Design review of the part built by this model. Coordinates are the model's own, in mm. Face numbers are marked on the shaded views. A direction names the side the tool comes from. Coordinates: 2 decimals unless noted, no trailing zeros. Loops run counter-clockwise (first coordinate to the right, second up) from the corner with the lowest first, then second, coordinate; pieces in that order, holes last. Notation, with made-up numbers: (60, 82) - (74, 82) arc R28 ccw to (74, 117) - close; hole circle Ø9 at (-34.75, -2). An arc over 180 degrees is marked (long way). Answer in a Markdown table with one row per item. Add a question column.
(1) We need section C-C, the plane z = -1.75. Write out the cut boundary in (x, y).
(2) We need section D-D, the plane x = 0. Write out the cut boundary in (y, z).
(3) The part is to be moulded in two halves that separate along Y. For the marked faces 3, 4, 5 and 6, say which applies: released by +Y, released by -Y, zero draft, split by the parting line, or undercut.
(4) We need section B-B, the plane x = -7.5. Write out the cut boundary in (y, z), plus the area to 3 significant figures.
(5) To check wall thickness, follow L1, parallel to Y at x = 24.5, z = -3; L2, parallel to X at y = -9.5, z = 2.75; L3, parallel to X at y = 12.5, z = 0. State the ranges of each line that lie inside material, in increasing order. Write a range as [from, to].
(6) Clearance check with a flat-ended pin moving along its axis: pin 1 (6.5 mm diameter, centred on x = 30, z = 0, fed in from -Y). State where the tip first meets the part, or that it passes through.
(7) For the marked faces 1 and 2, list the 3-axis set-ups (+Z, -Z, +X, -X, +Y, -Y) from which the entire face can be reached by the end or side of a thin tool; tool diameter is ignored.
(8) We need section A-A, the plane y = -4. Write out the cut boundary in (x, z), plus the area to 3 significant figures.
from build123d import *

# Parameters (mm, degrees)
F0_W          = 75
F0_H          = 50
F0_W_2        = 60
F0_H_2        = 40
F1_DEPTH      = 12.5
F2_R          = 2.5
F3_DEPTH      = 25.001
F3_DEPTH_BACK = 25.001


with BuildPart() as f1:
    # F0 (on Top) → F1 (new body, symmetric)
    with BuildSketch(Plane.XY):
        Rectangle(F0_W, F0_H)
        Rectangle(F0_W_2, F0_H_2, mode=Mode.SUBTRACT)
    extrude(amount=F1_DEPTH, both=True)

    # F2 (on Front) → F3 (cut, two sides)
    with BuildSketch(Plane.XZ) as f3_sk:
        with Locations((-30, 0)):
            Circle(F2_R)
        with Locations((30, 0)):
            Circle(F2_R)
        Circle(F2_R)
    extrude(amount=-F3_DEPTH, mode=Mode.SUBTRACT)
    extrude(f3_sk.sketch, amount=F3_DEPTH_BACK, mode=Mode.SUBTRACT)


solid = f1.part
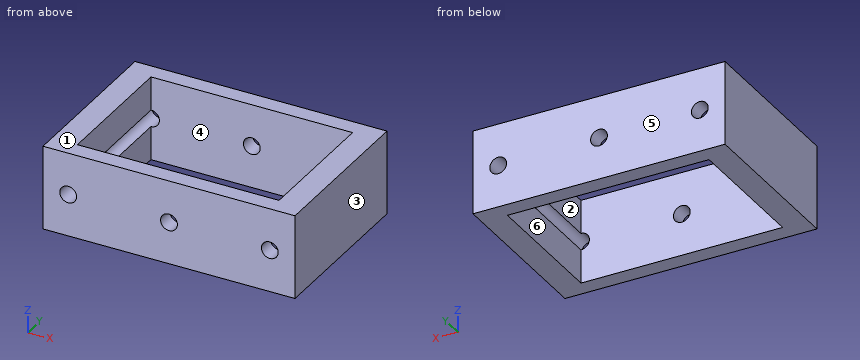
Responses:
| question | item | result |
|---|---|---|
| 1 | outline | (-37.5, -25) - (-31.79, -25) - (-31.79, 25) - (-37.5, 25) - close; (-28.21, -25) - (-1.79, -25) - (-1.79, -20) - (-28.21, -20) - close; (-28.21, 20) - (-1.79, 20) - (-1.79, 25) - (-28.21, 25) - close; (1.79, -25) - (28.21, -25) - (28.21, -20) - (1.79, -20) - close; (1.79, 20) - (28.21, 20) - (28.21, 25) - (1.79, 25) - close; (31.79, -25) - (37.5, -25) - (37.5, 25) - (31.79, 25) - close |
| 2 | outline | (-25, -12.5) - (-20, -12.5) - (-20, -2.5) - (-25, -2.5) - close; (-25, 2.5) - (-20, 2.5) - (-20, 12.5) - (-25, 12.5) - close; (20, -12.5) - (25, -12.5) - (25, -2.5) - (20, -2.5) - close; (20, 2.5) - (25, 2.5) - (25, 12.5) - (20, 12.5) - close |
| 3 | face 3 | zero draft |
| 3 | face 4 | undercut |
| 3 | face 5 | released by +Y |
| 3 | face 6 | undercut |
| 4 | outline | (-25, -12.5) - (-20, -12.5) - (-20, 12.5) - (-25, 12.5) - close; (20, -12.5) - (25, -12.5) - (25, 12.5) - (20, 12.5) - close |
| 4 | area | 250 mm2 |
| 5 | L1 | y = [-25, -20], [20, 25] |
| 5 | L2 | x = [-37.5, -30], [30, 37.5] |
| 5 | L3 | x = [-37.5, -32.5], [32.5, 37.5] |
| 6 | pin 1 | stops at y = -25 |
| 7 | face 1 | +Z, +X, -X, +Y, -Y |
| 7 | face 2 | +Z, -Z |
| 8 | outline | (-37.5, -12.5) - (-30, -12.5) - (-30, -2.5) arc R2.5 cw to (-30, 2.5) - (-30, 12.5) - (-37.5, 12.5) - close; (30, -12.5) - (37.5, -12.5) - (37.5, 12.5) - (30, 12.5) - (30, 2.5) arc R2.5 cw to (30, -2.5) - close |
| 8 | area | 355 mm2 |
